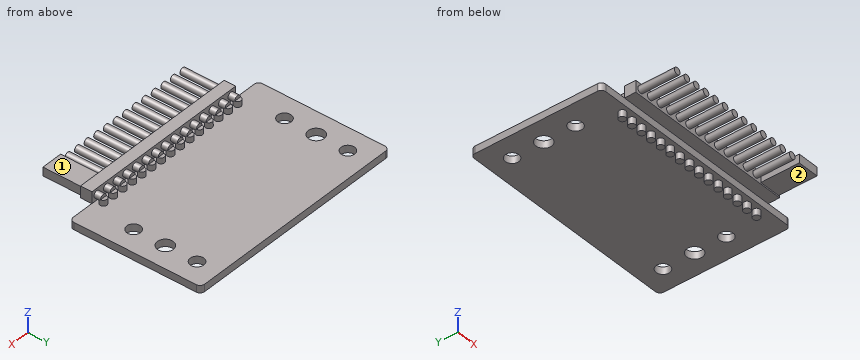
from build123d import *

# Parameters (mm, degrees)
F0_W      = 50
F0_H      = 29
F0_R      = 0.635
F0_R_2    = 1.5
F0_R_3    = 1.75
F1_DEPTH  = 1.6
F2_R      = 1
F3_R      = 0.75
F4_DEPTH  = 1.25
F5_DEPTH  = 3.05
F7_R      = 0.75
F8_DEPTH  = 12.1
F10_W     = 38.1
F10_H     = 2.54
F11_DEPTH = 2.54
F12_W     = 4.6887147206
F12_H     = 1.8870429106
F13_DEPTH = 8.5


with BuildPart() as f1:
    # F0 (on Top) → F1 (new body)
    with BuildSketch(Plane.XY):
        with Locations((25, 14.5)):
            Rectangle(F0_W, F0_H)
        with Locations((7.22, 1.5)):
            Circle(F0_R, mode=Mode.SUBTRACT)
        with Locations((9.76, 1.5)):
            Circle(F0_R, mode=Mode.SUBTRACT)
        with Locations((12.3, 1.5)):
            Circle(F0_R, mode=Mode.SUBTRACT)
        with Locations((14.84, 1.5)):
            Circle(F0_R, mode=Mode.SUBTRACT)
        with Locations((17.38, 1.5)):
            Circle(F0_R, mode=Mode.SUBTRACT)
        with Locations((19.92, 1.5)):
            Circle(F0_R, mode=Mode.SUBTRACT)
        with Locations((22.46, 1.5)):
            Circle(F0_R, mode=Mode.SUBTRACT)
        with Locations((5, 10)):
            Circle(F0_R_2, mode=Mode.SUBTRACT)
        with Locations((25, 1.5)):
            Circle(F0_R, mode=Mode.SUBTRACT)
        with Locations((27.54, 1.5)):
            Circle(F0_R, mode=Mode.SUBTRACT)
        with Locations((30.08, 1.5)):
            Circle(F0_R, mode=Mode.SUBTRACT)
        with Locations((32.62, 1.5)):
            Circle(F0_R, mode=Mode.SUBTRACT)
        with Locations((35.16, 1.5)):
            Circle(F0_R, mode=Mode.SUBTRACT)
        with Locations((37.7, 1.5)):
            Circle(F0_R, mode=Mode.SUBTRACT)
        with Locations((40.24, 1.5)):
            Circle(F0_R, mode=Mode.SUBTRACT)
        with Locations((42.78, 1.5)):
            Circle(F0_R, mode=Mode.SUBTRACT)
        with Locations((45, 10)):
            Circle(F0_R_2, mode=Mode.SUBTRACT)
        with Locations((5, 17)):
            Circle(F0_R_3, mode=Mode.SUBTRACT)
        with Locations((5, 24)):
            Circle(F0_R_2, mode=Mode.SUBTRACT)
        with Locations((45, 17)):
            Circle(F0_R_3, mode=Mode.SUBTRACT)
        with Locations((45, 24)):
            Circle(F0_R_2, mode=Mode.SUBTRACT)
    extrude(amount=F1_DEPTH)

    # F2
    f2_edges = [f1.edges().sort_by_distance(p)[0] for p in [
        (0, 0, 0.8),
        (50, 0, 0.8),
        (50, 29, 0.8),
        (0, 29, 0.8),
    ]]
    fillet(f2_edges, radius=F2_R)

    # F3 (on face) → F4 (join)
    with BuildSketch(Plane.XY.offset(1.6)):
        with Locations((9.76, 1.5)):
            Circle(F3_R)
        with Locations((12.3, 1.5)):
            Circle(F3_R)
        with Locations((14.84, 1.5)):
            Circle(F3_R)
        with Locations((17.38, 1.5)):
            Circle(F3_R)
        with Locations((19.92, 1.5)):
            Circle(F3_R)
        with Locations((22.46, 1.5)):
            Circle(F3_R)
        with Locations((25, 1.5)):
            Circle(F3_R)
        with Locations((27.54, 1.5)):
            Circle(F3_R)
        with Locations((30.08, 1.5)):
            Circle(F3_R)
        with Locations((32.62, 1.5)):
            Circle(F3_R)
        with Locations((35.16, 1.5)):
            Circle(F3_R)
        with Locations((37.7, 1.5)):
            Circle(F3_R)
        with Locations((40.24, 1.5)):
            Circle(F3_R)
        with Locations((42.78, 1.5)):
            Circle(F3_R)
        with Locations((7.22, 1.5)):
            Circle(F3_R)
    extrude(amount=F4_DEPTH)

    # F3 (on face) → F5 (join)
    with BuildSketch(Plane.XY.offset(1.6)):
        with Locations((9.76, 1.5)):
            Circle(F3_R)
        with Locations((12.3, 1.5)):
            Circle(F3_R)
        with Locations((14.84, 1.5)):
            Circle(F3_R)
        with Locations((17.38, 1.5)):
            Circle(F3_R)
        with Locations((19.92, 1.5)):
            Circle(F3_R)
        with Locations((22.46, 1.5)):
            Circle(F3_R)
        with Locations((25, 1.5)):
            Circle(F3_R)
        with Locations((27.54, 1.5)):
            Circle(F3_R)
        with Locations((30.08, 1.5)):
            Circle(F3_R)
        with Locations((32.62, 1.5)):
            Circle(F3_R)
        with Locations((35.16, 1.5)):
            Circle(F3_R)
        with Locations((37.7, 1.5)):
            Circle(F3_R)
        with Locations((40.24, 1.5)):
            Circle(F3_R)
        with Locations((42.78, 1.5)):
            Circle(F3_R)
        with Locations((7.22, 1.5)):
            Circle(F3_R)
    extrude(amount=-F5_DEPTH)

    # F7 (on offset) → F8 (join)
    with BuildSketch(Plane.XZ.offset(-1.5)):
        with Locations((9.76, 2.85)):
            Circle(F7_R)
        with Locations((12.3, 2.85)):
            Circle(F7_R)
        with Locations((14.84, 2.85)):
            Circle(F7_R)
        with Locations((17.38, 2.85)):
            Circle(F7_R)
        with Locations((19.92, 2.85)):
            Circle(F7_R)
        with Locations((22.46, 2.85)):
            Circle(F7_R)
        with Locations((25, 2.85)):
            Circle(F7_R)
        with Locations((27.54, 2.85)):
            Circle(F7_R)
        with Locations((30.08, 2.85)):
            Circle(F7_R)
        with Locations((32.62, 2.85)):
            Circle(F7_R)
        with Locations((35.16, 2.85)):
            Circle(F7_R)
        with Locations((37.7, 2.85)):
            Circle(F7_R)
        with Locations((40.24, 2.85)):
            Circle(F7_R)
        with Locations((42.78, 2.85)):
            Circle(F7_R)
        with Locations((7.22, 2.85)):
            Circle(F7_R)
    extrude(amount=F8_DEPTH)

    # F10 (on offset) → F11 (join)
    with BuildSketch(Plane.XZ.offset(2.52)):
        with Locations((25, 2.85)):
            Rectangle(F10_W, F10_H)
    extrude(amount=-F11_DEPTH)

    # F12 (on face) → F13 (join)
    with BuildSketch(Plane.XZ.offset(2.52)):
        with Locations((41.4229617903, 2.85)):
            Rectangle(F12_W, F12_H)
    extrude(amount=F13_DEPTH)


solid = f1.part
Read the model definition and answer for the solid it produces. Units are mm, in the model's axes. Face numbers are marked on the shaded views. A direction names the side the tool comes from. Coordinates: 2 decimals unless noted, no trailing zeros. Loops run counter-clockwise (first coordinate to the right, second up) from the corner with the lowest first, then second, coordinate; pieces in that order, holes last. Notation, with made-up numbers: (-0.75, 64) -> (53.25, 64) arc R5 ccw to (53.25, 69) -> close; hole circle Ø4 at (-2.75, -20). An arc over 180 degrees is marked (long way). Answer in a Markdown table with one row per item.
Item 1: A cutting plane is placed at C-C on z = 0.8. Determine the outline of the cut face in (x, y), plus the area to 3 significant figures.
Returned:
| item | result |
|---|---|
| outline | (0, 1) arc R1 ccw to (1, 0) -> (49, 0) arc R1 ccw to (50, 1) -> (50, 28) arc R1 ccw to (49, 29) -> (1, 29) arc R1 ccw to (0, 28) -> close; hole circle Ø3.5 at (5, 17); hole circle Ø3 at (5, 10); hole circle Ø3 at (5, 24); hole circle Ø3.5 at (45, 17); hole circle Ø3 at (45, 10); hole circle Ø3 at (45, 24) |
| area | 1,400 mm^2 |
Item 2: Straight lines are drawn through the part: line 1 along Y through (x, z) = (5, 0.95); line 2 along Y through (x, z) = (4.5, 1.1); line 3 along Z through (x, y) = (44, 3.5). For each, find the intervals that lie inside material, in ascending order. Write a range as [from, to].
Returned:
| item | result |
|---|---|
| line 1 | y = [0, 8.5], [11.5, 15.25], [18.75, 22.5], [25.5, 29] |
| line 2 | y = [0, 8.59], [11.41, 15.32], [18.68, 22.59], [25.41, 29] |
| line 3 | z = [0, 1.6] |
Item 3: For the marked faces 1 and 2, determine the directions among +Z, -Z, +X, -X, +Y, -Y from which every point of the face is accessible in a straight line to the end or side of a thin tool.
Returned:
| item | result |
|---|---|
| face 1 | +Z, +X, -X, -Y |
| face 2 | -Z, +X, -X, -Y |
Item 4: A cutting plane is placed at D-D on x = 9.76. Determine the outline of the cut face in (y, z), plus the area to 3 significant figures.
Returned:
| item | result |
|---|---|
| outline | (-10.6, 2.1) -> (-2.52, 2.1) -> (-2.52, 1.58) -> (0, 1.58) -> (0, 0) -> (0.75, 0) -> (0.75, -1.45) -> (2.25, -1.45) -> (2.25, 0) -> (29, 0) -> (29, 1.6) -> (2.25, 1.6) -> (2.25, 2.85) -> (1.5, 2.85) -> (1.5, 3.6) -> (0.02, 3.6) -> (0.02, 4.12) -> (-2.52, 4.12) -> (-2.52, 3.6) -> (-10.6, 3.6) -> close; hole (0.02, 1.6) -> (0.75, 1.6) -> (0.75, 2.1) -> (0.02, 2.1) -> close |
| area | 70.7 mm^2 |
Item 5: Each of these flat-tipped pins is pushed along its axis until it touches: P1, Ø0.8, axis at x = 12, z = 3.5, coming from the +Y side; P2, Ø0.8, axis at x = 9.5, z = 3, coming from the +Y side; P3, Ø14.5, axis at x = 31, y = 19.5, coming from the +Z side; P4, Ø3, axis at x = 25.5, z = 2, coming from the +Y side. Where does it stop, or does it pass through?
Returned:
| item | result |
|---|---|
| P1 | stops at y = 1.5 |
| P2 | stops at y = 2.25 |
| P3 | stops at z = 1.6 |
| P4 | stops at y = 29 |
Item 6: A cutting plane is placed at A-A on x = 45. Determine the outline of the cut face in (y, z).
Returned:
| item | result |
|---|---|
| outline | (0, 0) -> (8.5, 0) -> (8.5, 1.6) -> (0, 1.6) -> close; (11.5, 0) -> (15.25, 0) -> (15.25, 1.6) -> (11.5, 1.6) -> close; (18.75, 0) -> (22.5, 0) -> (22.5, 1.6) -> (18.75, 1.6) -> close; (25.5, 0) -> (29, 0) -> (29, 1.6) -> (25.5, 1.6) -> close |
Item 7: A cutting plane is placed at B-B on y = 17. Determine the outline of the cut face in (x, z).
Returned:
| item | result |
|---|---|
| outline | (0, 0) -> (3.25, 0) -> (3.25, 1.6) -> (0, 1.6) -> close; (6.75, 0) -> (43.25, 0) -> (43.25, 1.6) -> (6.75, 1.6) -> close; (46.75, 0) -> (50, 0) -> (50, 1.6) -> (46.75, 1.6) -> close |
